Part model, mm, in its own coordinate system. Face numbers are marked on the shaded views. A direction names the side the tool comes from. Round coordinates to 2 decimals unless told otherwise and drop trailing zeros. Order: outer loops, then holes, each group sorted by start corner. A loop starts at its lowest first (then second) coordinate and runs counter-clockwise, first axis right, second up. Notation, with made-up numbers: (53.25, -28.5) - (59.25, -28.5) arc R26 cw to (59.25, -6.5) - close; hole circle Ø11 at (-9.75, 6). An arc over 180 degrees is marked (long way). Return JSON: item names as keys, results as strings. Group by question number.
Item 1: Tool access for the marked faces 1, 2 and 3: list every direction of +Z, -Z, +X, -X, +Y, -Y with a clear straight run to the whole face (end or side of a thin tool).
Item 2: Two-plate mould, pull along Z, no slides. Class the marked faces 4, 5, 6 and 7: released by +Z, released by -Z, zero draft, split by the parting line, or undercut.
Item 3: Saw through at B-B on y = 1.75. List the corners of the cut face in (x, z).
Item 4: Probe probe 1 along Z at (x, y) = (-10.5, -2.5); probe 2 along Y at (x, z) = (10.5, 13.25) (3 decimals); probe 3 along X at (y, z) = (-1.75, 1). List the from-to ranges inside material, lowest first.
Item 5: Drop flat-ended pins along their axis: pin 1 (0.7 mm diameter, centred on y = 0.5, z = 3, fed in from +X); pin 2 (1 mm diameter, centred on y = 1, z = 15.5, fed in from +X); pin 3 (8 mm diameter, centred on x = 0.5, z = 13, fed in from +Y) (3 decimals); pin 4 (2 mm diameter, centred on x = -14, y = 0.5, fed in from -Z). Give the stop position or say it passes through.
Item 6: Saw through at C-C on x = 6. List the corners of the cut face in (y, z) (3 decimals), and give its area (3 significant figures).
Item 7: Saw through at A-A on z = 7.75. List the corners of the cut face in (x, y) (3 decimals).
```python
from build123d import *

# Parameters (mm, degrees)
F1_DEPTH = 3.75
F2_DEPTH = 2.125


with BuildPart() as f1:
    # F0 (on Front) → F1 (new body, symmetric)
    with BuildSketch(Plane.XZ):
        Polygon((-14.613904, 1.5), (-14.613904, 0), (14.686096, 0), (14.686096, 1.5), (13.186096, 1.5), (-13.213904, 1.5), align=None)
    extrude(amount=F1_DEPTH, both=True)

    # F0 (on Front) → F2 (join, symmetric)
    with BuildSketch(Plane.XZ):
        with BuildLine():
            Line((-13.213904, 3.75), (-13.213904, 1.5))
            Line((-13.213904, 1.5), (13.186096, 1.5))
            Line((13.186096, 1.5), (13.186096, 3.75))
            Line((13.186096, 3.75), (11.592854, 13.61754))
            Line((11.592854, 13.61754), (9.826933, 16.639381))
            Line((9.826933, 16.639381), (12.417082, 18.153027))
            ThreePointArc((12.417082, 18.153027), (13.11117, 19.067501), (12.955334, 20.204925))
            ThreePointArc((12.955334, 20.204925), (12.04086, 20.899013), (10.903436, 20.743177))
            Line((10.903436, 20.743177), (4.47028, 16.983732))
            ThreePointArc((4.47028, 16.983732), (4.014538, 16.399349), (4.086191, 15.661739))
            Line((4.086191, 15.661739), (10.071552, 4.064036))
            Line((10.071552, 4.064036), (8.877797, 3.366423))
            Line((8.877797, 3.366423), (1.711417, 14.273954))
            ThreePointArc((1.711417, 14.273954), (1.103954, 14.698445), (0.371112, 14.588236))
            Line((0.371112, 14.588236), (-14.470727, 5.914875))
            ThreePointArc((-14.470727, 5.914875), (-15.01491, 5.36638), (-15.213904, 4.6198))
            Line((-15.213904, 4.6198), (-15.213904, 3.75))
            Line((-15.213904, 3.75), (-13.213904, 3.75))
        make_face()
    extrude(amount=F2_DEPTH, both=True)


solid = f1.part
```
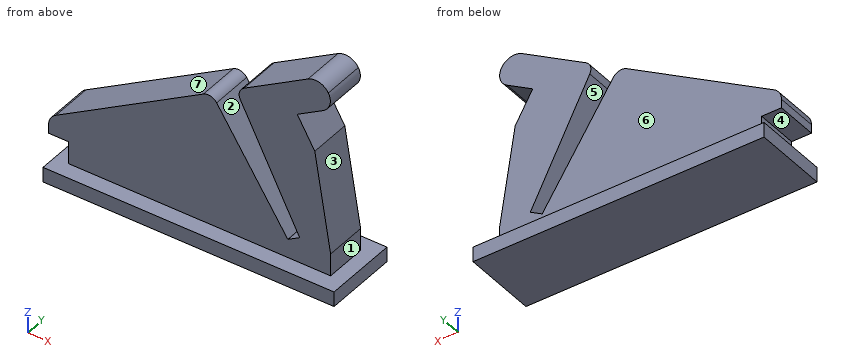
Filled in:
{
 "1": {"face 1": "+Z, +X, +Y, -Y", "face 2": "+Y, -Y", "face 3": "+X, +Y, -Y"},
 "2": {"face 4": "undercut", "face 5": "undercut", "face 6": "zero draft", "face 7": "released by +Z"},
 "3": {"outline": "(-15.21, 3.75) - (-13.21, 3.75) - (-13.21, 1.5) - (-14.61, 1.5) - (-14.61, 0) - (14.69, 0) - (14.69, 1.5) - (13.19, 1.5) - (13.19, 3.75) - (11.59, 13.62) - (9.83, 16.64) - (12.42, 18.15) arc R1.5 ccw to (10.9, 20.74) - (4.47, 16.98) arc R1 ccw to (4.09, 15.66) - (10.07, 4.06) - (8.88, 3.37) - (1.71, 14.27) arc R1 ccw to (0.37, 14.59) - (-14.47, 5.91) arc R1.5 ccw to (-15.21, 4.62) - close"},
 "4": {"probe 1": "z = 0 to 1.5", "probe 2": "y = -2.125 to 2.125", "probe 3": "x = -14.61 to 14.69"},
 "5": {"pin 1": "stops at x = 13.19", "pin 2": "stops at x = 10.78", "pin 3": "stops at y = 2.125", "pin 4": "stops at z = 0"},
 "6": {"outline": "(-3.75, 0) - (3.75, 0) - (3.75, 1.5) - (2.125, 1.5) - (2.125, 7.747) - (-2.125, 7.747) - (-2.125, 1.5) - (-3.75, 1.5) - close; (-2.125, 11.953) - (2.125, 11.953) - (2.125, 17.878) - (-2.125, 17.878) - close", "area": "63.0 mm^2"},
 "7": {"outline": "(-11.33, -2.125) - (5.998, -2.125) - (5.998, 2.125) - (-11.33, 2.125) - close; (8.169, -2.125) - (12.54, -2.125) - (12.54, 2.125) - (8.169, 2.125) - close"}
}
